Autodesk Inventor part; units mm, degrees
ref_plane "YZ Plane" through (0, 0, 0) normal (1, 0, 0) x (0, 1, 0)
ref_plane "XZ Plane" through (0, 0, 0) normal (0, 1, 0) x (-1, 0, 0)
ref_plane "XY Plane" through (0, 0, 0) normal (0, 0, 1) x (1, 0, 0)
sketch "Sketch1" plane through (0, 0, 0) normal (0, 1, 0) x (-1, 0, 0)
  line L0 (30, 45) -> (-30, 45)
  line L1 (-30, 45) -> (-30, -45)
  line L2 (-30, -45) -> (30, -45)
  line L3 (30, -45) -> (30, 45)
  line L4 (30, 45) -> (-30, -45) construction
  line L5 (-30, 45) -> (30, -45) construction
  point P0 (0, 0)
  dimension "d0" = 60
  dimension "d1" = 90
extrude "Extrusion1" add sketch "Sketch1" along normal blind 15
sketch "Sketch2" plane through (0, 15, 0) normal (0, 1, 0) x (1, 0, 0)
  line L0 (-30, 45) -> (-30, -45)
  line L1 (-30, 45) -> (-20, 45)
  line L2 (-20, 45) -> (-20, 39)
  line L3 (-20, 39) -> (-30, 39)
  line L4 (-30, 39) -> (-30, 45)
  line L5 (30, -45) -> (30, 45)
  line L6 (30, 45) -> (20, 45)
  line L7 (20, 45) -> (20, 39)
  line L8 (20, 39) -> (30, 39)
  line L9 (30, 39) -> (30, 45)
  line L10 (30, -45) -> (25.5, -45)
  line L11 (25.5, -45) -> (25.5, -29)
  line L12 (25.5, -29) -> (30, -29)
  line L13 (30, -29) -> (30, -45)
  line L14 (-30, -45) -> (-25, -45)
  line L15 (-25, -45) -> (-25, -29)
  line L16 (-25, -29) -> (-30, -29)
  line L17 (-30, -29) -> (-30, -45)
  line L18 (30, 45) -> (-30, 45)
  line L19 (-30, 45) -> (-24, 45)
  line L20 (-24, 45) -> (-24, 35)
  line L21 (-24, 35) -> (-30, 35)
  line L22 (-30, 35) -> (-30, 45)
  line L23 (30, 45) -> (24.316, 45)
  line L24 (24.316, 45) -> (24.316, 35)
  line L25 (24.316, 35) -> (30, 35)
  line L26 (30, 35) -> (30, 45)
  line L27 (-30, -45) -> (30, -45)
  line L28 (-30, -45) -> (-25.5, -45)
  line L29 (-25.5, -45) -> (-25.5, -29)
  line L30 (-25.5, -29) -> (-30, -29)
  line L31 (-30, -29) -> (-30, -45)
  point P0 (0, 0)
  dimension "d4" = 10
  dimension "d5" = 6
  dimension "d6" = 10
  dimension "d7" = 4.5
  dimension "d8" = 16
  dimension "d17" = 6
  dimension "d18" = 10
  dimension "d19" = 5.684
  dimension "d20" = 10
  dimension "d21" = 4.5
fillet "Fillet1" radius 4 2 edges at (30, 7.5, -45) (-30, 7.5, -45)
hole "Hole2" at (-24, 15, -35) at (24.316, 15, -35) at (25.5, 15, 29) at (-25.5, 15, 29) direction (0, -1, 0) diameter 5 end through all
ref_plane "Work Plane2" through (-30, 0, 35) normal (0, 0, 1) x (1, 0, 0)
sketch "Sketch3" plane through (-30, 0, 35) normal (0, 0, 1) x (1, 0, 0)
  line L0 (0, 15) -> (17.5, 15)
  line L1 (2, 15) -> (7, 15)
  line L2 (17.5, 15) -> (17.5, 17.5)
  line L3 (17.5, 17.5) -> (42.5, 17.5)
  circle A0 centre (42.5, 17.5) radius 5
  circle A1 centre (17.5, 17.5) radius 5
  point P0 (30, 0)
  dimension "d31" = 17.5
  dimension "d32" = 2.5
  dimension "d33" = 25
  dimension "d34" = 10
  dimension "d35" = 10
extrude "Extrusion2" cut sketch "Sketch3" against normal blind 15
fillet "Fillet2" radius 2 2 edges at (-12.5, 12.5, 20) (12.5, 12.5, 20)
properties part number "Adaptador_soporte_motor-rueda_error_asumido"
Could you check a few things on this model? Use its own coordinates, in mm. A direction names the side the tool comes from. Coordinates: 2 decimals unless noted, no trailing zeros. Loops run counter-clockwise (first coordinate to the right, second up) from the corner with the lowest first, then second, coordinate; pieces in that order, holes last. Notation, with made-up numbers: M 68,19.25 L 101,19.25 A35 ccw 101,58.25 Z; hole C 11,47 d1. An arc over 180 degrees is marked long. Put each result on its own line as item: value. Start each with the question number.
(1) I need wall thicknesses on line 1 (X direction, y = 6.5, z = -35); line 2 (X direction, y = 10.25, z = 29); line 3 (Z direction, x = -24, y = 4.25). Which ranges of each line are inside material? Lowest first, please. Write a range as from..to.
(2) Thinking about a two-plate mould opening in Z: for faces 1 (the face through (0, 7, -45)), 2 (the face through (0, 7, 45)), 3 (the face through (-26.11, 7.4, -33.66)), 4 (the face through (0, 15, 1)), which applies, pulls with the +Z half, pulls with the -Z half, needs draft (parallel to the pull), parting line crosses it, or undercut?
(3) For faces 5 (the face through (-13, 14, 35)), 6 (the face through (23, 7, 29)), which set-ups out of +Z, -Z, +X, -X, +Y, -Y let a thin tool reach every point of the face, with its end or its side?
(4) Will this pin go through, and if not, where does the flat tip stop? P1, Ø3, axis at x = 25.5, z = 29, coming from the -Y side.
(5) Suppose I cut it at C-C on y = 10.5. Please give me the cut outline in (x, z).
(6) Suppose I cut it at B-B on z = -35. Please give me the cut outline in (x, y), then the cut area to 3 significant figures.
(7) Suppose I cut it at A-A on x = -24. Please give me the cut outline in (y, z).
(8) Suppose I cut it at D-D on z = 29. Please give me the cut outline in (x, y), then the cut area to 3 significant figures.
Solutions:
1. line 1: x = -30..-26.5, -21.5..21.82, 26.82..30
1. line 2: x = -30..-28, -23..23, 28..30
1. line 3: z = -45..-37.5, -32.5..27, 31..45
2. face 1: pulls with the -Z half
2. face 2: pulls with the +Z half
2. face 3: undercut
2. face 4: needs draft
3. face 5: +Y
3. face 6: +Y, -Y
4. P1: passes through
5. outline: M -30,-41 A4 ccw -26,-45 L 26,-45 A4 ccw 30,-41 L 30,45 L -30,45 Z; hole C -25.5,29 d5; hole C -24,-35 d5; hole C 24.32,-35 d5; hole C 25.5,29 d5
6. outline: M -30,0 L -26.5,0 L -26.5,15 L -30,15 Z; M -21.5,0 L 21.82,0 L 21.82,15 L -21.5,15 Z; M 26.82,0 L 30,0 L 30,15 L 26.82,15 Z
6. area: 750 mm2
7. outline: M 0,-45 L 15,-45 L 15,-37.5 L 0,-37.5 Z; M 0,-32.5 L 15,-32.5 L 15,27 L 0,27 Z; M 0,31 L 15,31 L 15,45 L 0,45 Z
8. outline: M -30,0 L -28,0 L -28,15 L -30,15 Z; M -23,0 L 23,0 L 23,15 L 16.83,15 A5 cw 8.17,15 L -8.17,15 A5 cw -16.83,15 L -23,15 Z; M 28,0 L 30,0 L 30,15 L 28,15 Z
8. area: 719 mm2
